For this review, take the finished solid that the model builds, in its own axes (mm). Face numbers are marked on the shaded views. A direction names the side the tool comes from. Round coordinates to 2 decimals unless told otherwise and drop trailing zeros. Loops run counter-clockwise (first coordinate to the right, second up) from the corner with the lowest first, then second, coordinate; pieces in that order, holes last.
1) Tool access review of the marked faces 4, 5 and 6: name each direction out of +Z, -Z, +X, -X, +Y, -Y from which nothing blocks a thin tool from reaching the whole face with its end or side.
2) Take a section at C-C (x = 35). State the section outline as (y, z) points.
3) Take a section at D-D (z = 6.5). State the section outline as (x, y) points.
4) Take a section at A-A (y = -45). State the section outline as (x, z) points.
5) Mouldability with a two-part tool opening along X and no side actions: class the marked faces 1, 2 and 3 as pulls with the +X half, pulls with the -X half, needs draft (parallel to the pull), parting line crosses it, or undercut.
6) Take a section at B-B (y = -53). State the section outline as (x, z) points.
7) Insertion check: pin 1 (22 mm diameter, centred on x = 44.5, z = 13.5, fed in from -Y); pin 2 (1.5 mm diameter, centred on x = 30.5, y = -24.5, fed in from +Z) (3 decimals); pin 3 (10 mm diameter, centred on y = -17, z = 35.5, fed in from -X). Each pin has a flat end and moves straight along its axis. Give the tip position at first contact, or say it passes through.
8) Wall thickness on L1, parallel to X at y = -46.5, z = 13.5; L2, parallel to Y at x = 55, z = 11; L3, parallel to Y at x = 47, z = 49: over which ranges is each line inside the solid? List them lowest first.
```python
from build123d import *

# Parameters (mm, degrees)
F1_DEPTH = 95
F3_DEPTH = 10.001
F4_W     = 57
F4_H     = 24
F5_DEPTH = 25


with BuildPart() as f1:
    # F0 (on Right) → F1 (new body)
    with BuildSketch(Plane.YZ):
        Polygon((-60, 0), (0, 0), (0, 56), (-10, 56), (-10, 28), (-60, 13), align=None)
    extrude(amount=F1_DEPTH)

    # F2 (on face) → F3 (cut, through all)
    with BuildSketch(Plane.XZ.offset(10)):
        Polygon((55.181451, 56), (95, 28), (95, 56), align=None)
    extrude(amount=-F3_DEPTH, mode=Mode.SUBTRACT)

    # F4 (on face) → F5 (cut)
    with BuildSketch(Plane(origin=(0, 0, 0), x_dir=(1, 0, 0), z_dir=(0, 0, -1))):
        with Locations((47.5, 48)):
            Rectangle(F4_W, F4_H)
    extrude(amount=-F5_DEPTH, mode=Mode.SUBTRACT)


solid = f1.part
```
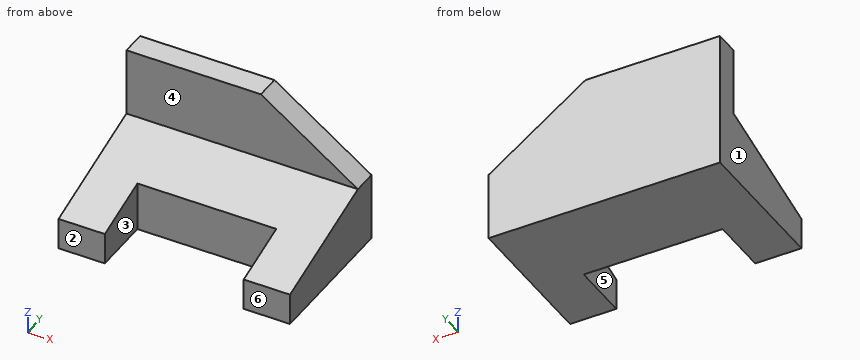
Response:
1. face 4: +Z, +X, -X, -Y
1. face 5: +Z, -Z, -Y
1. face 6: +Z, -Z, +X, -X, -Y
2. outline: (-36, 0) - (0, 0) - (0, 56) - (-10, 56) - (-10, 28) - (-36, 20.2) - close
3. outline: (0, -60) - (19, -60) - (19, -36) - (76, -36) - (76, -60) - (95, -60) - (95, 0) - (0, 0) - close
4. outline: (0, 0) - (19, 0) - (19, 17.5) - (0, 17.5) - close; (76, 0) - (95, 0) - (95, 17.5) - (76, 17.5) - close
5. face 1: pulls with the -X half
5. face 2: needs draft
5. face 3: undercut
6. outline: (0, 0) - (19, 0) - (19, 15.1) - (0, 15.1) - close; (76, 0) - (95, 0) - (95, 15.1) - (76, 15.1) - close
7. pin 1: stops at y = -36
7. pin 2: stops at z = 23.875
7. pin 3: passes through
8. L1: x = 0 to 19, 76 to 95
8. L2: y = -36 to 0
8. L3: y = -10 to 0
